Input: part model. Units: mm. Frame: model coordinates. Face numbers are marked on the shaded views. Coordinates: 2 decimals unless noted, no trailing zeros. Order: outer loops, then holes, each group sorted by start corner. A loop starts at its lowest first (then second) coordinate and runs counter-clockwise, first axis right, second up. Notation, with made-up numbers: (43, 59) -> (54, 59) arc R25 cw to (54, 95) -> close; hole circle Ø10 at (75.5, -34). An arc over 180 degrees is marked (long way). One line per question, with ' | ' between items.
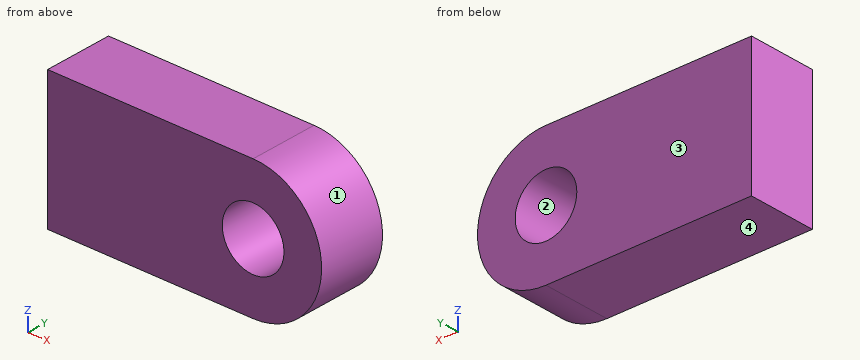
```python
from build123d import *

# Parameters (mm, degrees)
CYLINDER001_R     = 1.8
CYLINDER001_DEPTH = 30
CYLINDER_R        = 4
CYLINDER_DEPTH    = 4
BOX008_W          = 12
BOX008_H          = 4
BOX008_DEPTH      = 8


with BuildPart() as cylinder001:
    # Cylinder001 → Cylinder001 (new body)
    with BuildSketch(Plane(origin=(0, 0, 4), x_dir=(1, 0, 0), z_dir=(0, 1, 0))):
        Circle(CYLINDER001_R)
    extrude(amount=CYLINDER001_DEPTH)


with BuildPart() as cylinder:
    # Cylinder → Cylinder (new body)
    with BuildSketch(Plane(origin=(0, 0, 4), x_dir=(1, 0, 0), z_dir=(0, 1, 0))):
        Circle(CYLINDER_R)
    extrude(amount=CYLINDER_DEPTH)


with BuildPart() as ear:
    # Box008 → Box008 (new body)
    with BuildSketch(Plane.XY):
        with Locations((6, 2)):
            Rectangle(BOX008_W, BOX008_H)
    extrude(amount=BOX008_DEPTH)

    # Fusion: union Cylinder
    add(cylinder.part)

    # Cut: cut Cylinder001
    add(cylinder001.part, mode=Mode.SUBTRACT)


with BuildPart() as ear_1:
    # Cut placement: moved
    add(ear.part.moved(Location((-12, 51, -2))))


with BuildPart() as part_mirroring:
    # Part__Mirroring: instance of ear
    add(ear_1.part.mirror(Plane(origin=(32.4, 0, 0), x_dir=(0, -1, 0), z_dir=(1, 0, 0))))


solid = part_mirroring.part
```
1. Ray query, line 1 (X direction, y = 52.2, z = 2); line 2 (Z direction, x = 76.8, y = 54); line 3 (Z direction, x = 75.75, y = 52.45). Return the intervals inside material, ascending. Write a range as [from, to].
Recorded:
line 1: x = [64.8, 75], [78.6, 80.8] | line 2: z = [-2, 0.2], [3.8, 6] | line 3: z = [-2, 0.54], [3.46, 6]
2. Mould query, pull axis Z, two halves, no side actions, for the marked faces 1, 2, 3 and 4. Classes: released by +Z, released by -Z, zero draft, split by the parting line, or undercut.
Recorded:
face 1: split by the parting line | face 2: undercut | face 3: zero draft | face 4: released by -Z
3. Cut plane B-B, the plane y = 53.7. Return loops of the section in (x, z).
Recorded:
outline: (64.8, -2) -> (76.8, -2) arc R4 ccw to (76.8, 6) -> (64.8, 6) -> close; hole circle Ø3.6 at (76.8, 2)
4. Cut plane C-C, the plane x = 77.25. Return loops of the section in (y, z).
Recorded:
outline: (51, -1.97) -> (55, -1.97) -> (55, 0.26) -> (51, 0.26) -> close; (51, 3.74) -> (55, 3.74) -> (55, 5.97) -> (51, 5.97) -> close
5. Pin query (flat end, axial travel): pin 1 Ø1.5 at (y, z) = (53, 3.5) entering from +X. Return the tip coordinate at first contact, or that it passes through.
Recorded:
pin 1: stops at x = 80.73
6. Cut plane A-A, the plane z = 2. Return loops of the section in (x, y).
Recorded:
outline: (64.8, 51) -> (75, 51) -> (75, 55) -> (64.8, 55) -> close; (78.6, 51) -> (80.8, 51) -> (80.8, 55) -> (78.6, 55) -> close
